Geometry: final body of the model. Coordinates: model frame, mm. A direction names the side the tool comes from. Round coordinates to 2 decimals unless told otherwise and drop trailing zeros. Order: outer loops, then holes, each group sorted by start corner. A loop starts at its lowest first (then second) coordinate and runs counter-clockwise, first axis right, second up. Notation, with made-up numbers: (41.5, 48) -> (93.5, 48) arc R17 ccw to (93.5, 73) -> close; hole circle Ø5 at (24.25, -30). An arc over 180 degrees is marked (long way). Put each result on its own line as item: value.
```python
from build123d import *

# Parameters (mm, degrees)
CHAMFER1_SIZE                   = 8.89
F_5_32_0_15625_DIAMETER_HOLE1_D = 3.96875


with BuildPart() as part:
    # Sketch1 → Revolve1 (revolve)
    with BuildSketch(Plane.XY, mode=Mode.PRIVATE) as revolve1_sk:
        Polygon((-29.337, 0), (-41.275, 0), (-41.275, -9.525), (0, -9.525), (0, 0), (-21.1455, 0), (-21.1455, 9.525), (-29.337, 9.525), align=None)
    revolve(revolve1_sk.sketch.rotate(Axis((0, -9.525, 0), (0, 1, 0)), 270), axis=Axis((0, -9.525, 0), (0, 1, 0)))

    # Chamfer1
    chamfer1_edges = [part.edges().sort_by_distance(p)[0] for p in [
        (0, -9.525, 41.275),
    ]]
    chamfer(chamfer1_edges, length=CHAMFER1_SIZE)

    # 5/32 (0.15625) Diameter Hole1 (through all)
    with Locations(Plane(origin=(0, -9.525, 0), x_dir=(0, 0, -1), z_dir=(0, -1, 0))):
        with Locations((0, 0)):
            Hole(F_5_32_0_15625_DIAMETER_HOLE1_D / 2)


solid = part.part
```
1. Material intervals for probe 1 along X at (y, z) = (6, 0); probe 2 along Y at (x, z) = (5.5, -2) (3 decimals); probe 3 along Z at (x, y) = (-1.5, 4.5), sorted ascending.
Ans:
probe 1: -29.34 to -21.15, 21.15 to 29.34
probe 2: -9.525 to 0
probe 3: -29.3 to -21.09, 21.09 to 29.3
2. Cut plane A-A on z = 0. Return loops of the section in (x, y) (1 decimal), and give its area (4 significant figures).
Ans:
outline: (-41.3, -0.6) -> (-32.4, -9.5) -> (-2, -9.5) -> (-2, 0) -> (-21.1, 0) -> (-21.1, 9.5) -> (-29.3, 9.5) -> (-29.3, 0) -> (-41.3, 0) -> close; (2, -9.5) -> (32.4, -9.5) -> (41.3, -0.6) -> (41.3, 0) -> (29.3, 0) -> (29.3, 9.5) -> (21.1, 9.5) -> (21.1, 0) -> (2, 0) -> close
area: 825.5 mm²
3. Cut plane C-C on y = 1.75. Return loops of the section in (x, z).
Ans:
outline: circle Ø58.67 at (0, 0); hole circle Ø42.29 at (0, 0)
4. Contact query for flat-ended pins moving along their axis: P1, Ø1, axis at x = -22.5, y = -1.5, coming from the -Z side; P2, Ø3, axis at y = 1, z = 10.5, coming from the +X side; P3, Ø2, axis at y = 3, z = 22.5, coming from the -X side. Output: stop coordinate, or through.
Ans:
P1: z = -34.25
P2: x = 40.19
P3: x = -19.96
5. Cut plane B-B on x = 0. Return loops of the section in (y, z) (1 decimal).
Ans:
outline: (-9.5, -32.4) -> (-0.6, -41.3) -> (0, -41.3) -> (0, -29.3) -> (9.5, -29.3) -> (9.5, -21.1) -> (0, -21.1) -> (0, -2) -> (-9.5, -2) -> close; (-9.5, 2) -> (0, 2) -> (0, 21.1) -> (9.5, 21.1) -> (9.5, 29.3) -> (0, 29.3) -> (0, 41.3) -> (-0.6, 41.3) -> (-9.5, 32.4) -> close
6. Set-up query: faces 1 (the face through (-29.087, 4.696, 3.819)), 2 (the face through (-40.924, -0.322, 5.373)). Return all of +Z, -Z, +X, -X, +Y, -Y with unobstructed straight access to the full face (end or side cutting, diameter ignored); none if empty.
Ans:
face 1: +Y
face 2: +Y, -Y
7. Cut plane D-D on y = -3.5. Return loops of the section in (x, z).
Ans:
outline: circle Ø76.82 at (0, 0); hole circle Ø3.97 at (0, 0)
